Part model, mm, in its own coordinate system. A direction names the side the tool comes from. Round coordinates to 2 decimals unless told otherwise and drop trailing zeros. Loops run counter-clockwise (first coordinate to the right, second up) from the corner with the lowest first, then second, coordinate; pieces in that order, holes last. Notation, with made-up numbers: (7, 48) -> (12, 48) arc R19 ccw to (12, 77) -> close; hole circle Ø7 at (12, 68). An arc over 180 degrees is marked (long way). Answer as CSV lines item,"result".
from build123d import *

# Parameters (mm, degrees)
BOSS_EXTRUDE1_DEPTH = 36.45
FILLET1_R           = 5
FILLET2_R           = 20
SHELL2_T            = -1.2
BOSS_EXTRUDE2_START = 2
SKETCH3_R           = 1.5
BOSS_EXTRUDE2_DEPTH = 2
SKETCH4_W           = 3
SKETCH4_H           = 39.083354503
BOSS_EXTRUDE3_DEPTH = 13
FILLET3_R           = 10
CUT_EXTRUDE1_DEPTH  = 13


with BuildPart() as part:
    # Sketch1 → Boss-Extrude1 (new body)
    with BuildSketch(Plane.XY):
        with BuildLine():
            Line((-72.731515082, -496.215408036), (-35.731515082, -496.215408036))
            Line((-35.731515082, -496.215408036), (-35.731515082, -592.831160904))
            Line((-35.731515082, -592.831160904), (-47.731515082, -592.831160904))
            Line((-47.731515082, -592.831160904), (-47.731515082, -598.627239774))
            Line((-47.731515082, -598.627239774), (-80.731515082, -598.627239774))
            Line((-80.731515082, -598.627239774), (-80.731515082, -504.215408036))
            ThreePointArc((-80.731515082, -504.215408036), (-78.388369332, -498.558553786), (-72.731515082, -496.215408036))
        make_face()
    extrude(amount=BOSS_EXTRUDE1_DEPTH)

    # Fillet1
    fillet1_edges = [part.edges().sort_by_distance(p)[0] for p in [
        (-47.731515082, -592.831160904, 18.225),
    ]]
    fillet(fillet1_edges, radius=FILLET1_R)

    # Fillet2
    fillet2_edges = [part.edges().sort_by_distance(p)[0] for p in [
        (-39.231515082, -592.831160904, 36.45),
        (-46.267048988, -594.295626999, 36.45),
        (-47.731515082, -598.229200339, 36.45),
    ]]
    fillet(fillet2_edges, radius=FILLET2_R)

    # Shell2
    shell2_openings = [part.faces().sort_by_distance(p)[0] for p in [
        (-78.388369332, -498.558553786, 18.225),
        (-80.731515082, -551.421323905, 18.225),
        (-65.156208184, -598.627239774, 17.167742853),
        (-35.731515082, -543.427965052, 17.881276605),
        (-54.231515082, -496.215408036, 18.225),
        (-58.408271611, -546.88462098, 0),
    ]]
    offset(amount=SHELL2_T, openings=shell2_openings, kind=Kind.INTERSECTION)

    # Sketch3 → Boss-Extrude2 (add)
    with BuildSketch(Plane.XY.offset(8).offset(BOSS_EXTRUDE2_START)):
        with BuildLine():
            Line((-47.731515082, -597.831160904), (-47.731515082, -600.270500733))
            Line((-47.731515082, -600.270500733), (-43.792175254, -600.270500733))
            ThreePointArc((-43.792175254, -600.270500733), (-41.31730152, -599.245374467), (-40.292175254, -596.770500733))
            Line((-40.292175254, -596.770500733), (-40.292175254, -592.831160904))
            Line((-40.292175254, -592.831160904), (-42.731515082, -592.831160904))
            ThreePointArc((-42.731515082, -592.831160904), (-46.267048988, -594.295626999), (-47.731515082, -597.831160904))
        make_face()
        with Locations((-43.792175254, -596.770500733)):
            Circle(SKETCH3_R, mode=Mode.SUBTRACT)
    extrude(amount=-BOSS_EXTRUDE2_DEPTH)

    # Sketch4 → Boss-Extrude3 (add)
    with BuildSketch(Plane.XY.offset(36.45)):
        with Locations((-60.045293953, -539.622953905)):
            Rectangle(SKETCH4_W, SKETCH4_H)
    extrude(amount=BOSS_EXTRUDE3_DEPTH)

    # Fillet3
    fillet3_edges = [part.edges().sort_by_distance(p)[0] for p in [
        (-60.045293953, -559.164631156, 49.45),
        (-60.045293953, -520.081276653, 49.45),
    ]]
    fillet(fillet3_edges, radius=FILLET3_R)

    # Sketch5 → Cut-Extrude1 (cut)
    with BuildSketch(Plane(origin=(-58.545293953, 0, 0), x_dir=(0, 0, -1), z_dir=(1, 0, 0))):
        with BuildLine():
            Line((-39.45, -556.164631156), (-39.45, -523.081276653))
            ThreePointArc((-39.45, -523.081276653), (-44.399747468, -525.131529185), (-46.45, -530.081276653))
            Line((-46.45, -530.081276653), (-46.45, -549.164631156))
            ThreePointArc((-46.45, -549.164631156), (-44.399747468, -554.114378625), (-39.45, -556.164631156))
        make_face()
    extrude(amount=-CUT_EXTRUDE1_DEPTH, mode=Mode.SUBTRACT)


solid = part.part
Q1. Saw through at C-C, the plane z = 4.5. Write the cut outline in (x, y).
Geometry results:
outline,"(-48.93, -598.63) -> (-47.73, -598.63) -> (-47.73, -597.83) arc R5 cw to (-42.73, -592.83) -> (-35.73, -592.83) -> (-35.73, -591.63) -> (-42.73, -591.63) arc R6.2 ccw to (-48.93, -597.83) -> close"
Q2. Saw through at B-B, the plane z = 42.5. Write the cut outline in (x, y).
Geometry results:
outline,"(-61.55, -558.69) -> (-58.55, -558.69) -> (-58.55, -555.47) -> (-61.55, -555.47) -> close; (-61.55, -523.78) -> (-58.55, -523.78) -> (-58.55, -520.56) -> (-61.55, -520.56) -> close"
Q3. Drill centre lines: line 1 along Z through (x, y) = (-48.5, -517); line 2 along X through (y, z) = (-558, 37); line 3 along Y through (x, z) = (-41, 14.5). Where is each one in solid material? Low to high.
Geometry results:
line 1,"35.25 to 36.45"
line 2,"-61.55 to -58.55"
line 3,"-592.83 to -591.63"
Q4. Two-plate mould, pull along Y, no slides. Class faces 5 (the face through (-60.024, -556.313, 46.443)), 6 (the face through (-60.02, -525.08, 44.35)), 7 (the face through (-60, -539, 49.45)): pulls with the +Y half, pulls with the -Y half, needs draft (parallel to the pull), parting line crosses it, or undercut.
Geometry results:
face 5,"pulls with the -Y half"
face 6,"undercut"
face 7,"needs draft"
Q5. Drop flat-ended pins along their axis: P1, Ø1, axis at x = -62, y = -589.5, coming from the +Z side; P2, Ø10, axis at x = -53.5, y = -541.5, coming from the +Z side; P3, Ø0.6, axis at y = -598, z = 10.5, coming from the -X side; P4, Ø1.8, axis at x = -43.79, y = -596.77, coming from the -Z side. Give the stop position or say it passes through.
Geometry results:
P1,"z = 36.14"
P2,"z = 36.45"
P3,"x = -48.93"
P4,"through"
Q6. Saw through at D-D, the plane x = -39. Write the cut outline in (y, z).
Geometry results:
outline,"(-592.83, 0) -> (-591.63, 0) -> (-591.63, 16.45) arc R18.8 cw to (-572.83, 35.25) -> (-496.22, 35.25) -> (-496.22, 36.45) -> (-572.83, 36.45) arc R20 ccw to (-592.83, 16.45) -> close"
Q7. Saw through at A-A, the plane y = -547. Write the cut outline in (x, z).
Geometry results:
outline,"(-80.73, 35.25) -> (-35.73, 35.25) -> (-35.73, 36.45) -> (-58.55, 36.45) -> (-58.55, 39.45) -> (-61.55, 39.45) -> (-61.55, 36.45) -> (-80.73, 36.45) -> close; (-61.55, 46.45) -> (-58.55, 46.45) -> (-58.55, 49.45) -> (-61.55, 49.45) -> close"
Q8. Which spindle directions (+Z, -Z, +X, -X, +Y, -Y) get a long thin tool onto all of the face, cutting with end or side? Do faces 1 (the face through (-46.23, -594.26, 4.06)), 2 (the face through (-40.292, -595, 9)), 3 (the face through (-46.23, -594.26, 13.27)), 4 (the face through (-60.024, -554.06, 44.454)). Say none if no direction does.
Geometry results:
face 1,"-Z, +X, -Y"
face 2,"+Z, -Z, +X, -Y"
face 3,"+Z, +X, -Y"
face 4,"+X, -X"
